```python
from build123d import *

# Parameters (mm, degrees)
BOSS_EXTRUDE2_START  = 1250
BOSS_EXTRUDE2_DEPTH  = 20
SKETCH3_W            = 20
SKETCH3_H            = 20
BOSS_EXTRUDE3_DEPTH  = 1250
LPATTERN1_COUNT      = 2
LPATTERN1_PITCH      = 840
MIRROR1_START        = 1250
MIRROR1_COPY_1_DEPTH = 20
SKETCH6_W            = 20
SKETCH6_H            = 20
BOSS_EXTRUDE7_DEPTH  = 730
SKETCH7_W            = 20
SKETCH7_H            = 379.823005399
BOSS_EXTRUDE8_DEPTH  = 20
CUT_EXTRUDE2_DEPTH   = 20
SKETCH10_W           = 20
SKETCH10_H           = 305.156338733
BOSS_EXTRUDE9_DEPTH  = 20
SKETCH11_W           = 150
SKETCH11_H           = 20
CUT_EXTRUDE3_DEPTH   = 20
BOSS_EXTRUDE10_DEPTH = 20


with BuildPart() as part:
    # Sketch2 → Boss-Extrude2 (new body)
    with BuildSketch(Plane(origin=(0, 0, 0), x_dir=(0, 0, -1), z_dir=(1, 0, 0)).offset(BOSS_EXTRUDE2_START)):
        Polygon((-2.643274402, -0.352436587), (-750, -100), (-750, -400), (-730, -400), (-730, -117.510327934), (0, -20.176994601), (0, 0), align=None)
    boss_extrude2 = extrude(amount=-BOSS_EXTRUDE2_DEPTH)

    # Sketch3 → Boss-Extrude3 (add, symmetric)
    with BuildSketch(Plane(origin=(0, 0, 0), x_dir=(0, 0, -1), z_dir=(1, 0, 0))):
        Polygon((0, -20.176994601), (-2.643274402, -0.352436587), (-22.467832415, -2.995710989), (-19.824558014, -22.820269002), align=None)
        with Locations((-740, -390)):
            Rectangle(SKETCH3_W, SKETCH3_H)
        with Locations((-740, -110)):
            Rectangle(SKETCH3_W, SKETCH3_H)
    extrude(amount=BOSS_EXTRUDE3_DEPTH, both=True)

    # LPattern1: Boss-Extrude2 ×2
    with Locations(*[(-i * LPATTERN1_PITCH, 0, 0) for i in range(1, LPATTERN1_COUNT)]):
        add(boss_extrude2)

    # Mirror1: Boss-Extrude2 across plane
    add(boss_extrude2.mirror(Plane(origin=(0, 0, 0), x_dir=(0, 0, 1), z_dir=(1, 0, 0))))

    # Mirror1 copy 1 sketch → Mirror1 copy 1 (add)
    with BuildSketch(Plane(origin=(840, 0, 0), x_dir=(0, 0, -1), z_dir=(-1, 0, 0)).offset(MIRROR1_START)):
        Polygon((-2.643274402, 0.352436587), (-750, 100), (-750, 400), (-730, 400), (-730, 117.510327934), (0, 20.176994601), (0, 0), align=None)
    extrude(amount=-MIRROR1_COPY_1_DEPTH)

    # Sketch6 → Boss-Extrude7 (add, through all)
    with BuildSketch(Plane(origin=(0, 0, 730), x_dir=(-1, 0, 0), z_dir=(0, 0, -1))):
        with Locations((-400, -390)):
            Rectangle(SKETCH6_W, SKETCH6_H)
        with Locations((400, -390)):
            Rectangle(SKETCH6_W, SKETCH6_H)
        with Locations((-1240, -390)):
            Rectangle(SKETCH6_W, SKETCH6_H)
        with Locations((1240, -390)):
            Rectangle(SKETCH6_W, SKETCH6_H)
    extrude(amount=BOSS_EXTRUDE7_DEPTH)

    # Sketch7 → Boss-Extrude8 (add)
    with BuildSketch(Plane(origin=(0, 0, 0), x_dir=(-1, 0, 0), z_dir=(0, 0, -1))):
        with Locations((-1240, -210.0884973)):
            Rectangle(SKETCH7_W, SKETCH7_H)
        with Locations((-400, -210.0884973)):
            Rectangle(SKETCH7_W, SKETCH7_H)
        with Locations((400, -210.0884973)):
            Rectangle(SKETCH7_W, SKETCH7_H)
        with Locations((1240, -210.0884973)):
            Rectangle(SKETCH7_W, SKETCH7_H)
    extrude(amount=-BOSS_EXTRUDE8_DEPTH)

    # Sketch9 → Cut-Extrude2 (cut)
    with BuildSketch(Plane.ZY.offset(1250)):
        Polygon((0, -400), (730, -400), (730, -117.510327934), (20, -22.843661267), (0, -20.176994601), align=None)
    extrude(amount=-CUT_EXTRUDE2_DEPTH, mode=Mode.SUBTRACT)

    # Sketch10 → Boss-Extrude9 (add)
    with BuildSketch(Plane(origin=(1250, 0, 0), x_dir=(0, 0, -1), z_dir=(1, 0, 0))):
        with Locations((-570, -247.421830634)):
            Rectangle(SKETCH10_W, SKETCH10_H)
    extrude(amount=-BOSS_EXTRUDE9_DEPTH)

    # Sketch11 → Cut-Extrude3 (cut)
    with BuildSketch(Plane(origin=(1250, 0, 0), x_dir=(0, 0, -1), z_dir=(1, 0, 0))):
        with Locations((-655, -390)):
            Rectangle(SKETCH11_W, SKETCH11_H)
    extrude(amount=-CUT_EXTRUDE3_DEPTH, mode=Mode.SUBTRACT)

    # Sketch12 → Boss-Extrude10 (add)
    with BuildSketch(Plane.ZY.offset(1250)):
        Polygon((0, -20.176994601), (20, -20.176994601), (20, -380), (560, -380), (560, -94.843661267), (580, -94.843661267), (580, -400), (0, -400), align=None)
    extrude(amount=-BOSS_EXTRUDE10_DEPTH)


solid = part.part
```
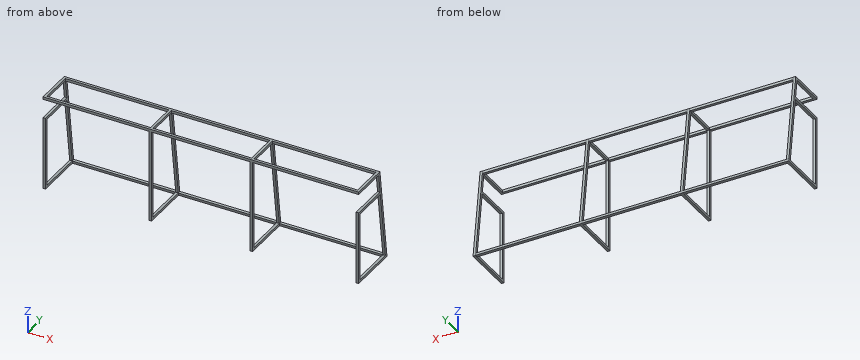
The listing builds one solid part. Answer for the finished solid, in the listing's coordinates (mm). Coordinates: 2 decimals unless noted, no trailing zeros. Write each loop counter-clockwise with the first axis right and the second up, starting at its lowest first coordinate (ties: lowest second). Pieces come first, ordered by that corner, then holes. Notation, with made-up numbers: (82.5, 64) -> (122.5, 64) arc R31 cw to (122.5, 99) -> close; hole circle Ø6 at (37.25, 70). An arc over 180 degrees is marked (long way). Write each question's results on one line, items separated by ' | '. Start each with the question number.
1) A cutting plane is placed at A-A (x = 220.5). Determine the outline of the cut face in (y, z), then the cut area to 3 significant figures.
2) A flat-ended cylindrical pin translates along its axis: pin 1 Ø10 at (x, z) = (-809.5, 744.5) entering from +Y. Find the tip coordinate at first contact, or state that the pin passes through.
3) A cutting plane is placed at C-C (y = -51). Count the separate pieces of the cut face and the enclosed holes in it, then the cut area to 3 significant figures.
4) A cutting plane is placed at B-B (z = 636). Determine the outline of the cut face in (x, y), then the cut area to 3 significant figures.
5) Straight lines are drawn through the part: probe 1 along X at (y, z) = (-89, 665); probe 2 along Z at (x, y) = (355.5, -382.5). For each, find the intervals that lie inside material, in ascending order.
Values follow:
1) outline: (-400, 730) -> (-380, 730) -> (-380, 750) -> (-400, 750) -> close; (-120, 730) -> (-100, 730) -> (-100, 750) -> (-120, 750) -> close; (-22.82, 19.82) -> (-20.18, 0) -> (-0.35, 2.64) -> (-3, 22.47) -> close | area: 1,200 mm²
2) pin 1: y = -100
3) separate pieces: 8 | enclosed holes: 0 | area: 13,700 mm²
4) outline: (-1250, -104.98) -> (-1230, -104.98) -> (-1230, -84.8) -> (-1250, -84.8) -> close; (-410, -400) -> (-390, -400) -> (-390, -380) -> (-410, -380) -> close; (-410, -104.98) -> (-390, -104.98) -> (-390, -84.8) -> (-410, -84.8) -> close; (390, -400) -> (410, -400) -> (410, -380) -> (390, -380) -> close; (390, -104.98) -> (410, -104.98) -> (410, -84.8) -> (390, -84.8) -> close; (1230, -104.98) -> (1250, -104.98) -> (1250, -84.8) -> (1230, -84.8) -> close | area: 2,410 mm²
5) probe 1: -1250 to -1230, -410 to -390, 390 to 410, 1230 to 1250 | probe 2: 730 to 750
